Design review of the part built by this model. Coordinates are the model's own, in mm. A direction names the side the tool comes from. Coordinates: 2 decimals unless noted, no trailing zeros. Loops run counter-clockwise (first coordinate to the right, second up) from the corner with the lowest first, then second, coordinate; pieces in that order, holes last.
Q1. Add section B-B on z = 0. Give the boundary of the cut face in (x, y).
Q2. Add section D-D on y = -3.5. Give the number of separate pieces and of enclosed holes in the cut face, and give its area (3 significant figures).
Q3. Wall thickness on probe 1 along X at (y, z) = (-1.5, 0); probe 2 along Z at (x, y) = (-18, -2.5); probe 3 along Z at (x, y) = (-2, -1.25): over which ranges is each line inside the solid? List them lowest first.
Q4. For P1, Ø6.5, axis at x = -1.59, z = -21.91, coming from the -Y side; P2, Ø2, axis at y = -5.5, z = 13, coming from the +X side; P3, Ø1.8, axis at x = -16.5, y = -3, coming from the -Z side, all flat-tipped, find the tip position at first contact; note any pin that passes through.
Q5. Add section C-C on z = -24. Give the boundary of the cut face in (x, y), and give its area (3 significant figures).
Q6. Add section A-A on x = 18. Give the boundary of the cut face in (y, z).
Q7. Machinability: for faces 4 (the face through (-4.206, -3.131, 15.606)), 5 (the face through (18, 0, -6)), which of the approach directions +Z, -Z, +X, -X, +Y, -Y give a long, thin tool a straight path to every point of the face, cutting with its end or side? Answer none if there is none.
Q8. Draft analysis for pull direction X (two halves, no side actions). For faces 1 (the face through (41.8, -3.13, 18.11)), 2 (the face through (1.51, -3.13, 4.81)), 3 (the face through (-8.572, -3, -20)), state which applies: released by +X, released by -X, zero draft, split by the parting line, or undercut.
```python
from build123d import *

# Parameters (mm, degrees)
SKETCH4_R           = 5.04
SKETCH4_R_2         = 3.96875
SKETCH4_R_3         = 2
SKETCH4_R_4         = 1.7272
BOSS_EXTRUDE2_DEPTH = 6.35


with BuildPart() as part:
    # Sketch4 → Boss-Extrude2 (new body)
    with BuildSketch(Plane(origin=(0, 0, 0), x_dir=(1, 0, 0), z_dir=(0, 1, 0))):
        with BuildLine():
            Line((40.257702493, -18.4375), (22.483900583, -18.4375))
            ThreePointArc((22.483900583, -18.4375), (21.500464498, -18.308390309), (20.583679925, -17.929811531))
            Line((20.583679925, -17.929811531), (10.779476649, -12.288263354))
            ThreePointArc((10.779476649, -12.288263354), (9.307944036, -11.804768953), (7.765559219, -11.946980575))
            Line((7.765559219, -11.946980575), (-16.517810325, -19.369406885))
            ThreePointArc((-16.517810325, -19.369406885), (-20.348558836, -18.710969534), (-22.098, -15.24))
            Line((-22.098, -15.24), (-22.098, 4.987500122))
            ThreePointArc((-22.098, 4.987500122), (-20.982076836, 7.681576958), (-18.288, 8.797500122))
            Line((-18.288, 8.797500122), (-12.3825, 8.797500122))
            ThreePointArc((-12.3825, 8.797500122), (-9.688423164, 9.913423286), (-8.5725, 12.607500122))
            Line((-8.5725, 12.607500122), (-8.5725, 26.9875))
            ThreePointArc((-8.5725, 26.9875), (-7.456576836, 29.681576836), (-4.7625, 30.7975))
            Line((-4.7625, 30.7975), (52.3875, 30.7975))
            ThreePointArc((52.3875, 30.7975), (55.081576836, 29.681576836), (56.1975, 26.9875))
            Line((56.1975, 26.9875), (56.1975, 19.362095927))
            ThreePointArc((56.1975, 19.362095927), (55.797199918, 17.662082259), (54.680415238, 16.319294633))
            Line((54.680415238, 16.319294633), (48.985566477, 12.027918285))
            ThreePointArc((48.985566477, 12.027918285), (47.868781798, 10.685130659), (47.468481715, 8.985116992))
            Line((47.468481715, 8.985116992), (47.468481715, -10.980610773))
            ThreePointArc((47.468481715, -10.980610773), (47.203372649, -12.376980446), (46.444939319, -13.579024524))
            Line((46.444939319, -13.579024524), (43.044160097, -17.225913752))
            ThreePointArc((43.044160097, -17.225913752), (41.776936446, -18.121498883), (40.257702493, -18.4375))
        make_face()
        with Locations(Location((0, 0, 0), (0, 0, 270))):
            Circle(SKETCH4_R, mode=Mode.SUBTRACT)
        with Locations(Location((-1.5875, 21.9075, 0), (0, 0, 270))):
            Circle(SKETCH4_R_2, mode=Mode.SUBTRACT)
        with Locations(Location((49.2125, 21.9075, 0), (0, 0, 270))):
            Circle(SKETCH4_R_2, mode=Mode.SUBTRACT)
        with Locations(Location((24.012521227, -14.703599027, 0), (0, 0, 270))):
            Circle(SKETCH4_R_3, mode=Mode.SUBTRACT)
        with Locations(Location((-17.78, -15.24, 0), (0, 0, 270))):
            Circle(SKETCH4_R_3, mode=Mode.SUBTRACT)
        with Locations(Location((18.000000004, 0, 0), (0, 0, 270))):
            Circle(SKETCH4_R_4, mode=Mode.SUBTRACT)
        with Locations(Location((-18.000000004, 0, 0), (0, 0, 270))):
            Circle(SKETCH4_R_4, mode=Mode.SUBTRACT)
    extrude(amount=-BOSS_EXTRUDE2_DEPTH)


solid = part.part
```
Entries:
1. outline: (-22.1, -6.35) - (-19.73, -6.35) - (-19.73, 0) - (-22.1, 0) - close; (-16.27, -6.35) - (-5.04, -6.35) - (-5.04, 0) - (-16.27, 0) - close; (5.04, -6.35) - (16.27, -6.35) - (16.27, 0) - (5.04, 0) - close; (19.73, -6.35) - (47.47, -6.35) - (47.47, 0) - (19.73, 0) - close
2. separate pieces: 1
2. enclosed holes: 7
2. area: 2,910 mm2
3. probe 1: x = -22.1 to -19.73, -16.27 to -5.04, 5.04 to 16.27, 19.73 to 47.47
3. probe 2: z = -8.8 to -1.73, 1.73 to 13.25, 17.23 to 19.55
3. probe 3: z = -30.8 to -25.85, -17.96 to -4.63, 4.63 to 14.93
4. P1: passes through
4. P2: stops at x = 47.33
4. P3: stops at z = -8.8
5. outline: (-8.57, -6.35) - (-4.96, -6.35) - (-4.96, 0) - (-8.57, 0) - close; (1.78, -6.35) - (45.84, -6.35) - (45.84, 0) - (1.78, 0) - close; (52.58, -6.35) - (56.2, -6.35) - (56.2, 0) - (52.58, 0) - close
5. area: 326 mm2
6. outline: (-6.35, -30.8) - (0, -30.8) - (0, -1.73) - (-6.35, -1.73) - close; (-6.35, 1.73) - (0, 1.73) - (0, 16.44) - (-6.35, 16.44) - close
7. face 4: +Z, +Y, -Y
7. face 5: +Z, -Z, +X, -X, +Y
8. face 1: released by +X
8. face 2: undercut
8. face 3: released by -X
